Part model, mm, in its own coordinate system. A direction names the side the tool comes from. Give positions to 0.01 mm unless a question says otherwise; leave off trailing zeros. Order: outer loops, then holes, each group sorted by start corner. A loop starts at its lowest first (then second) coordinate and runs counter-clockwise, first axis right, second up. Notation, with made-up numbers: (78.25, 49) - (123.25, 49) arc R24 ccw to (123.25, 82) - close; hole circle Ø5 at (-27.5, -9). An arc over 180 degrees is marked (long way). One line per item, written item: value.
```python
from build123d import *

# Parameters (mm, degrees)
F1_DEPTH = 8
F2_R     = 35
F3_DEPTH = 3
F4_R     = 8
F5_DEPTH = 37
F7_DEPTH = 136


# Not quite as in the source:
# - a feature names something its author has since deleted; it is built from what else it names


with BuildPart() as f1:
    # F0 (on Top) → F1 (new body)
    with BuildSketch(Plane.XY):
        with BuildLine():
            Line((-20.6155281281, 40), (-35, 40))
            ThreePointArc((-35, 40), (-38.5355339059, 38.5355339059), (-40, 35))
            Line((-40, 35), (-40, 20.6155281281))
            ThreePointArc((-40, 20.6155281281), (-37.348673038, 25.1013271024), (-34.1965616575, 29.25055847))
            ThreePointArc((-34.1965616575, 29.25055847), (-34.2946788875, 34.2946788875), (-29.25055847, 34.1965616575))
            ThreePointArc((-29.25055847, 34.1965616575), (-25.1013271024, 37.348673038), (-20.6155281281, 40))
        make_face()
        with BuildLine():
            ThreePointArc((-34.1965616575, 29.25055847), (-37.348673038, 25.1013271024), (-40, 20.6155281281))
            Line((-40, 20.6155281281), (-40, -20.6155281281))
            ThreePointArc((-40, -20.6155281281), (-37.348673038, -25.1013271024), (-34.1965616575, -29.25055847))
            ThreePointArc((-34.1965616575, -29.25055847), (-33.0960568151, -28.5607897045), (-31.8198051534, -28.3198051534))
            Line((-31.8198051534, -28.3198051534), (-31.8198051534, 28.3198051534))
            ThreePointArc((-31.8198051534, 28.3198051534), (-33.0960568151, 28.5607897045), (-34.1965616575, 29.25055847))
        make_face()
        with BuildLine():
            Line((28.3198051534, 31.8198051534), (-28.3198051534, 31.8198051534))
            ThreePointArc((-28.3198051534, 31.8198051534), (-29.3449314192, 29.3449314192), (-31.8198051534, 28.3198051534))
            Line((-31.8198051534, 28.3198051534), (-31.8198051534, -28.3198051534))
            ThreePointArc((-31.8198051534, -28.3198051534), (-29.3449314192, -29.3449314192), (-28.3198051534, -31.8198051534))
            ThreePointArc((-28.3198051534, -31.8198051534), (-28.5607897045, -33.0960568151), (-29.25055847, -34.1965616575))
            ThreePointArc((-29.25055847, -34.1965616575), (-25.1013271024, -37.348673038), (-20.6155281281, -40))
            Line((-20.6155281281, -40), (20.6155281281, -40))
            ThreePointArc((20.6155281281, -40), (25.1013271024, -37.348673038), (29.25055847, -34.1965616575))
            ThreePointArc((29.25055847, -34.1965616575), (29.3449314192, -29.3449314192), (34.1965616575, -29.25055847))
            ThreePointArc((34.1965616575, -29.25055847), (37.348673038, -25.1013271024), (40, -20.6155281281))
            Line((40, -20.6155281281), (40, 20.6155281281))
            ThreePointArc((40, 20.6155281281), (37.348673038, 25.1013271024), (34.1965616575, 29.25055847))
            ThreePointArc((34.1965616575, 29.25055847), (30.417779434, 28.612887025), (28.3198051534, 31.8198051534))
        make_face()
        with BuildLine():
            Line((20.6155281281, 40), (-20.6155281281, 40))
            ThreePointArc((-20.6155281281, 40), (-25.1013271024, 37.348673038), (-29.25055847, 34.1965616575))
            ThreePointArc((-29.25055847, 34.1965616575), (-28.5607897045, 33.0960568151), (-28.3198051534, 31.8198051534))
            Line((-28.3198051534, 31.8198051534), (28.3198051534, 31.8198051534))
            ThreePointArc((28.3198051534, 31.8198051534), (28.5607897045, 33.0960568151), (29.25055847, 34.1965616575))
            ThreePointArc((29.25055847, 34.1965616575), (25.1013271024, 37.348673038), (20.6155281281, 40))
        make_face()
        with BuildLine():
            Line((35, 40), (20.6155281281, 40))
            ThreePointArc((20.6155281281, 40), (25.1013271024, 37.348673038), (29.25055847, 34.1965616575))
            ThreePointArc((29.25055847, 34.1965616575), (33.0960568151, 35.0788206023), (35.3198051534, 31.8198051534))
            ThreePointArc((35.3198051534, 31.8198051534), (35.0267232818, 30.417779434), (34.1965616575, 29.25055847))
            ThreePointArc((34.1965616575, 29.25055847), (37.348673038, 25.1013271024), (40, 20.6155281281))
            Line((40, 20.6155281281), (40, 35))
            ThreePointArc((40, 35), (38.5355339059, 38.5355339059), (35, 40))
        make_face()
        with BuildLine():
            ThreePointArc((-34.1965616575, -29.25055847), (-37.348673038, -25.1013271024), (-40, -20.6155281281))
            Line((-40, -20.6155281281), (-40, -35))
            ThreePointArc((-40, -35), (-38.5355339059, -38.5355339059), (-35, -40))
            Line((-35, -40), (-20.6155281281, -40))
            ThreePointArc((-20.6155281281, -40), (-25.1013271024, -37.348673038), (-29.25055847, -34.1965616575))
            ThreePointArc((-29.25055847, -34.1965616575), (-34.2946788875, -34.2946788875), (-34.1965616575, -29.25055847))
        make_face()
        with BuildLine():
            Line((40, -35), (40, -20.6155281281))
            ThreePointArc((40, -20.6155281281), (37.348673038, -25.1013271024), (34.1965616575, -29.25055847))
            ThreePointArc((34.1965616575, -29.25055847), (35.0267232818, -30.417779434), (35.3198051534, -31.8198051534))
            ThreePointArc((35.3198051534, -31.8198051534), (33.0960568151, -35.0788206023), (29.25055847, -34.1965616575))
            ThreePointArc((29.25055847, -34.1965616575), (25.1013271024, -37.348673038), (20.6155281281, -40))
            Line((20.6155281281, -40), (35, -40))
            ThreePointArc((35, -40), (38.5355339059, -38.5355339059), (40, -35))
        make_face()
    extrude(amount=F1_DEPTH)

    # F2 (on face) → F3 (join)
    with BuildSketch(Plane(origin=(0, 0, 0), x_dir=(1, 0, 0), z_dir=(0, 0, -1))):
        Circle(F2_R)
    extrude(amount=F3_DEPTH)

    # F4 (on face) → F5 (join)
    with BuildSketch(Plane(origin=(0, 0, -3), x_dir=(1, 0, 0), z_dir=(0, 0, -1))):
        Circle(F4_R)
    extrude(amount=F5_DEPTH)

    # F6 (on face) → F7 (join)
    with BuildSketch(Plane.XY.offset(8)):
        with BuildLine():
            Line((-30.75, 25.75), (-38, 25.75))
            ThreePointArc((-38, 25.75), (-39.4142135624, 25.1642135624), (-40, 23.75))
            Line((-40, 23.75), (-40, -23.75))
            ThreePointArc((-40, -23.75), (-39.4142135624, -25.1642135624), (-38, -25.75))
            Line((-38, -25.75), (-30.75, -25.75))
            ThreePointArc((-30.75, -25.75), (-27.2144660941, -27.2144660941), (-25.75, -30.75))
            Line((-25.75, -30.75), (-25.75, -38))
            ThreePointArc((-25.75, -38), (-25.1642135624, -39.4142135624), (-23.75, -40))
            Line((-23.75, -40), (23.75, -40))
            ThreePointArc((23.75, -40), (25.1642135624, -39.4142135624), (25.75, -38))
            Line((25.75, -38), (25.75, -30.75))
            ThreePointArc((25.75, -30.75), (27.2144660941, -27.2144660941), (30.75, -25.75))
            Line((30.75, -25.75), (38, -25.75))
            ThreePointArc((38, -25.75), (39.4142135624, -25.1642135624), (40, -23.75))
            Line((40, -23.75), (40, 23.75))
            ThreePointArc((40, 23.75), (39.4142135624, 25.1642135624), (38, 25.75))
            Line((38, 25.75), (30.75, 25.75))
            ThreePointArc((30.75, 25.75), (27.2144660941, 27.2144660941), (25.75, 30.75))
            Line((25.75, 30.75), (25.75, 38))
            ThreePointArc((25.75, 38), (25.1642135624, 39.4142135624), (23.75, 40))
            Line((23.75, 40), (-23.75, 40))
            ThreePointArc((-23.75, 40), (-25.1642135624, 39.4142135624), (-25.75, 38))
            Line((-25.75, 38), (-25.75, 30.75))
            ThreePointArc((-25.75, 30.75), (-27.2144660941, 27.2144660941), (-30.75, 25.75))
        make_face()
    extrude(amount=F7_DEPTH)


solid = f1.part
```
1) Slice it at D-D on x = 11. Write the cut outline in (y, z).
Answer:
outline: (-40, 0) - (-33.23, 0) - (-33.23, -3) - (33.23, -3) - (33.23, 0) - (40, 0) - (40, 144) - (-40, 144) - close
2) Slice it at A-A on z = 96. Write the cut outline in (x, y), then the cut area to 3 significant figures.
Answer:
outline: (-40, -23.75) arc R2 ccw to (-38, -25.75) - (-30.75, -25.75) arc R5 cw to (-25.75, -30.75) - (-25.75, -38) arc R2 ccw to (-23.75, -40) - (23.75, -40) arc R2 ccw to (25.75, -38) - (25.75, -30.75) arc R5 cw to (30.75, -25.75) - (38, -25.75) arc R2 ccw to (40, -23.75) - (40, 23.75) arc R2 ccw to (38, 25.75) - (30.75, 25.75) arc R5 cw to (25.75, 30.75) - (25.75, 38) arc R2 ccw to (23.75, 40) - (-23.75, 40) arc R2 ccw to (-25.75, 38) - (-25.75, 30.75) arc R5 cw to (-30.75, 25.75) - (-38, 25.75) arc R2 ccw to (-40, 23.75) - close
area: 5,600 mm2
3) Slice it at B-B on x = 0. Write the cut outline in (y, z).
Answer:
outline: (-40, 0) - (-35, 0) - (-35, -3) - (-8, -3) - (-8, -40) - (8, -40) - (8, -3) - (35, -3) - (35, 0) - (40, 0) - (40, 144) - (-40, 144) - close
4) Two-plate mould, pull along X, no slides. Class faces 4 (the face through (-34, 25.75, 75)), 5 (the face through (-27.25, -27.18, 75.05)), 6 (the face through (38, -39, 4)): pulls with the +X half, pulls with the -X half, needs draft (parallel to the pull), parting line crosses it, or undercut.
Answer:
face 4: needs draft
face 5: pulls with the -X half
face 6: pulls with the +X half
5) Drop flat-ended pins along their axis: P1, Ø8, axis at x = 33.5, z = 76.5, coming from the -Y side; P2, Ø3.5, axis at y = -35.5, z = 91, coming from the +X side; P3, Ø2, axis at y = -36, z = 104, coming from the -X side. Give the stop position or say it passes through.
Answer:
P1: stops at y = -25.91
P2: stops at x = 25.75
P3: stops at x = -25.75
6) Which spindle directions (+Z, -Z, +X, -X, +Y, -Y) get a long thin tool onto all of the face, cutting with end or side? Do faces 1 (the face through (34, 25.75, 75)), 2 (the face through (35, -34, 8)), 3 (the face through (-25.75, -34, 75)). Say none if no direction does.
Answer:
face 1: +Z, +X, +Y
face 2: +Z, +X, -Y
face 3: +Z, -X, -Y
7) Wall check: line 1 along Y through (x, z) = (32, 3); line 2 along Z through (x, y) = (27.5, -12); line 3 along Z through (x, y) = (10.5, 34). Give the ranges that are in metal, low to high. Write a range as [from, to].
Answer:
line 1: y = [-40, -35.32], [-28.32, 28.32], [35.32, 40]
line 2: z = [-3, 144]
line 3: z = [0, 144]
